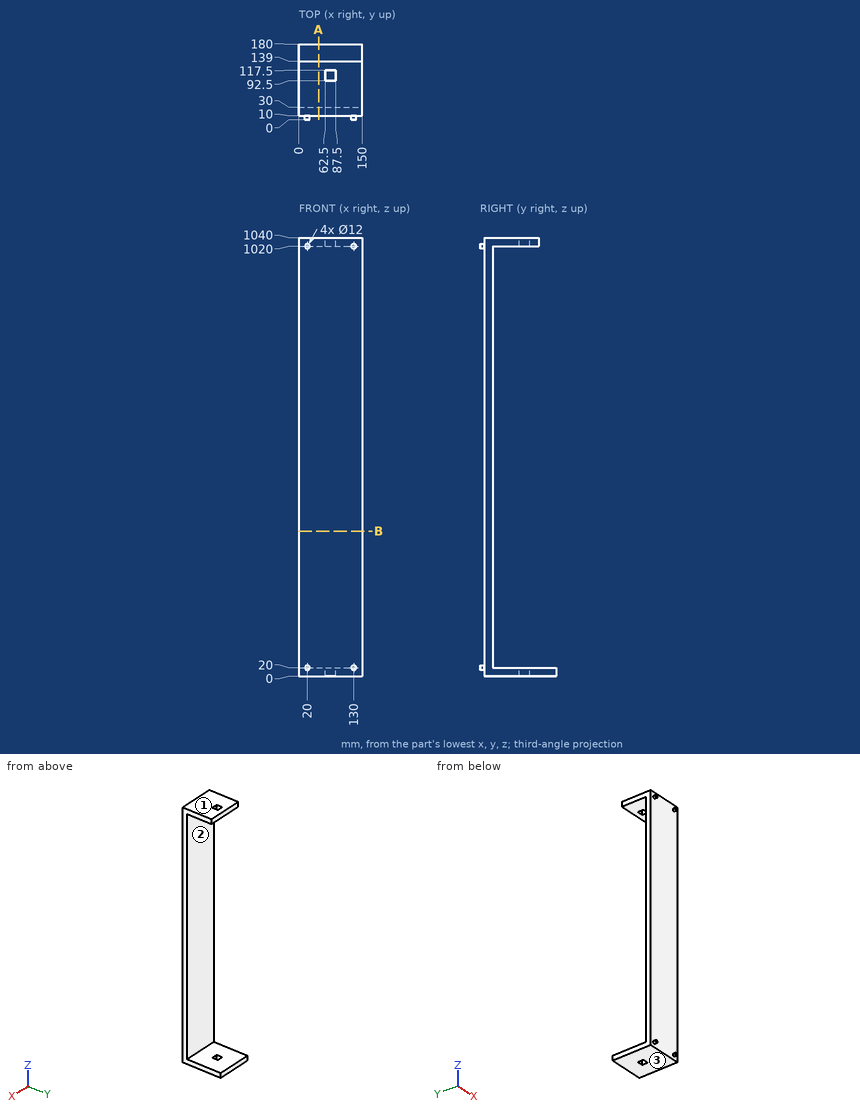
Could you check a few things on this drawing? It's one solid part, dimensions in mm from its lowest x, y, z. Round coordinates to 2 decimals unless told otherwise and drop trailing zeros. Order: outer loops, then holes, each group sorted by start corner. A loop starts at its lowest first (then second) coordinate and runs counter-clockwise, first axis right, second up. Notation, with made-up numbers: M 43,18.25 L 98,18.25 A18 cw 98,38.25 Z; hole C -17,82.25 d8. An arc over 180 degrees is marked long. Return JSON: item names as keys, results as strings. Group by question number.
1. If we section it at B-B on z = 344: List the corners of the cut face in (x, y) for me.
2. If we mould it in two halves opening along Z, with no side actions, what happens to the marked faces 1, 2 and 3? For each: pulls with the +Z half, pulls with the -Z half, needs draft (parallel to the pull), parting line crosses it, or undercut.
3. If we section it at A-A on x = 46.5: List the corners of the cut face in (y, z) for me.
4. Please list where these lines run through material, in increasing order: probe 1 along Z at (x, y) = (6.5, 40.5); probe 2 along Y at (x, z) = (111, 73.5); probe 3 along Z at (x, y) = (138.5, 154).
5. I'm going to push flat-ended pins straight in: pin 1 Ø6 at (x, z) = (49.5, 405.5) entering from -Y; pin 2 Ø6 at (x, z) = (74, 1029.5) entering from +Y; pin 3 Ø3 at (x, z) = (101.5, 413.5) entering from +Y. Where does each tip first touch, or does it pass through?
Reply:
{
 "1": {"outline": "M 0,10 L 150,10 L 150,30 L 0,30 Z"},
 "2": {"face 1": "pulls with the +Z half", "face 2": "undercut", "face 3": "pulls with the -Z half"},
 "3": {"outline": "M 10,0 L 180,0 L 180,20 L 30,20 L 30,1020 L 139,1020 L 139,1040 L 10,1040 Z"},
 "4": {"probe 1": "0 to 20, 1020 to 1040", "probe 2": "10 to 30", "probe 3": "0 to 20"},
 "5": {"pin 1": "y = 10", "pin 2": "y = 139", "pin 3": "y = 30"}
}
